Can you work these out from the model? Positions are in its coordinate system, mm. Give positions to 0.01 mm unless a question says otherwise; leave off trailing zeros. Loops run counter-clockwise (first coordinate to the right, second up) from the corner with the lowest first, then second, coordinate; pieces in that order, holes last. Notation, with made-up numbers: (-7.75, 74) - (7.25, 74) arc R19 cw to (7.25, 88) - close; hole circle Ø1 at (30, 12.25). An arc over 180 degrees is marked (long way). Answer in a Markdown table with one row per item.
from build123d import *

# Parameters (mm, degrees)
SKETCH1_R                 = 50
EXTRUDE1_DEPTH            = 5
M5_5_5_5_DIAMETER_HOLE2_D = 5.5


with BuildPart() as part:
    # Sketch1 → Extrude1 (new body)
    with BuildSketch(Plane.XY):
        Circle(SKETCH1_R)
    extrude(amount=-EXTRUDE1_DEPTH)

    # M5.5 (5.5) Diameter Hole2 (through all)
    with Locations(Plane.XY):
        with Locations((-31.819805153, 31.819805153), (31.819805153, 31.819805153), (31.819805153, -31.819805153), (-31.819805153, -31.819805153)):
            Hole(M5_5_5_5_DIAMETER_HOLE2_D / 2)


solid = part.part
Q1. Imagine slicing it at B-B, the plane z = -1.4. Write out the boundary of the cut face in (x, y), and give its area (3 significant figures).
Checked values:
| item | result |
|---|---|
| outline | circle Ø100 at (0, 0); hole circle Ø5.5 at (-31.82, -31.82); hole circle Ø5.5 at (-31.82, 31.82); hole circle Ø5.5 at (31.82, -31.82); hole circle Ø5.5 at (31.82, 31.82) |
| area | 7,760 mm² |
Q2. If we mould it in two halves opening along X, with no side actions, what happens to faces 1 (the face through (-1, 1, 0)), 2 (the face through (47.69, 15.02, -2.46)), 3 (the face through (29.28, -32.87, -2.53))? For each: released by +X, released by -X, zero draft, split by the parting line, or undercut.
Checked values:
| item | result |
|---|---|
| face 1 | zero draft |
| face 2 | split by the parting line |
| face 3 | undercut |
Q3. Imagine slicing it at A-A, the plane y = 33. Write out the boundary of the cut face in (x, z), and give its area (3 significant figures).
Checked values:
| item | result |
|---|---|
| outline | (-37.56, -5) - (-34.3, -5) - (-34.3, 0) - (-37.56, 0) - close; (-29.34, -5) - (29.34, -5) - (29.34, 0) - (-29.34, 0) - close; (34.3, -5) - (37.56, -5) - (37.56, 0) - (34.3, 0) - close |
| area | 326 mm² |
Q4. For pin 1 (5 mm diameter, centred on x = -31.82, y = 31.82, fed in from -Z); pin 2 (2 mm diameter, centred on y = 28.5, z = -3.5, fed in from +X); pin 3 (2 mm diameter, centred on x = -7.5, z = -2, fed in from -Y); pin 4 (1 mm diameter, centred on y = -29.5, z = -3.5, fed in from +X), each with a flat end and sliding along its axis, tell me the tip position at first contact or that it passes through.
Checked values:
| item | result |
|---|---|
| pin 1 | passes through |
| pin 2 | stops at x = 41.76 |
| pin 3 | stops at y = -49.58 |
| pin 4 | stops at x = 40.73 |
Q5. Imagine slicing it at D-D, the plane y = -15. Write out the boundary of the cut face in (x, z), and give its area (3 significant figures).
Checked values:
| item | result |
|---|---|
| outline | (-47.7, -5) - (47.7, -5) - (47.7, 0) - (-47.7, 0) - close |
| area | 477 mm² |
Q6. Imagine slicing it at C-C, the plane x = 37. Write out the boundary of the cut face in (y, z).
Checked values:
| item | result |
|---|---|
| outline | (-33.63, -5) - (33.63, -5) - (33.63, 0) - (-33.63, 0) - close |
Q7. If I drill on line 1 (Y direction, x = -33, z = -1.15); line 2 (Y direction, x = 0.5, z = -1), over which ranges is the centre line in solid material (lowest first)? Write a range as [from, to].
Checked values:
| item | result |
|---|---|
| line 1 | y = [-37.56, -34.3], [-29.34, 29.34], [34.3, 37.56] |
| line 2 | y = [-50, 50] |
